The listing builds one solid part. Answer for the finished solid, in the listing's coordinates (mm). Give positions to 0.01 mm unless a question says otherwise; leave off trailing zeros. Loops run counter-clockwise (first coordinate to the right, second up) from the corner with the lowest first, then second, coordinate; pieces in that order, holes last. Notation, with made-up numbers: M 62,67 L 82,67 A17 ccw 82,81 Z; hole C 26,16.25 d7. An arc over 180 degrees is marked long. One line per item, written item: value. Start each with the question number.
Q1. A cutting plane is placed at A-A, the plane y = 0. Determine the outline of the cut face in (x, z), and give its area (3 significant figures).
Q2. Flat-ended cylindrical pins translate along their axes: pin 1 (8 mm diameter, centred on x = 8.5, y = -2, fed in from -Z); pin 2 (1.8 mm diameter, centred on y = -1, z = -98, fed in from +X). Find the tip coordinate at first contact, or state that the pin passes through.
Q3. A cutting plane is placed at B-B, the plane z = -99. Determine the outline of the cut face in (x, y), and give its area (3 significant figures).
Q4. A cutting plane is placed at C-C, the plane x = 10. Determine the outline of the cut face in (y, z).
Q5. A cutting plane is placed at D-D, the plane z = -65.5. Determine the outline of the cut face in (x, y), and give its area (3 significant figures).
Q6. Consider L1, parallel to Y at x = 10, z = -50; L2, parallel to Y at x = 18.9, z = -99; L3, parallel to X at y = -0.5, z = -48. Determine where each line is inside the solid, lowest interval first.
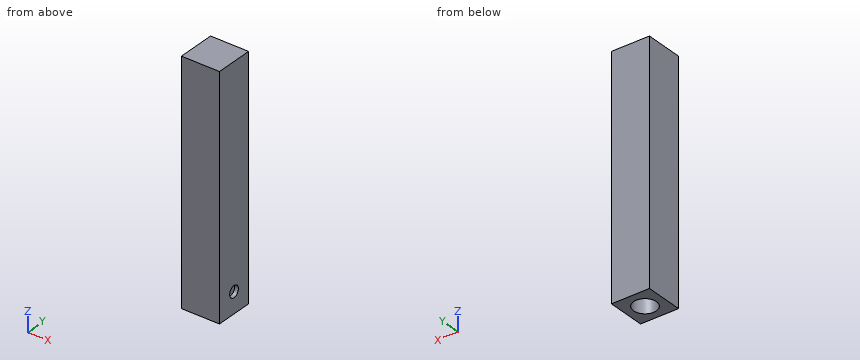
from build123d import *

# Parameters (mm, degrees)
EXTRUDE_1_DEPTH     = 20
SKETCH_2_R          = 6
CUT_EXTRUDE_1_DEPTH = 80
SKETCH_3_R          = 3
CUT_EXTRUDE_2_DEPTH = 2


with BuildPart() as part:
    # 草图1 → 凸台-拉伸1 (new body)
    with BuildSketch(Plane(origin=(0, 0, 0), x_dir=(0, 0, -1), z_dir=(1, 0, 0))):
        Polygon((-14.17593604, 10), (-14.175953417, -10), (110, -10), (110, 10), align=None)
    extrude(amount=EXTRUDE_1_DEPTH)

    # 草图2 → 切除-拉伸1 (cut)
    with BuildSketch(Plane(origin=(0, 0, -110), x_dir=(-1, 0, 0), z_dir=(0, 0, -1))):
        with Locations((-10, 0)):
            Circle(SKETCH_2_R)
    extrude(amount=-CUT_EXTRUDE_1_DEPTH, mode=Mode.SUBTRACT)

    # 草图3 → 切除-拉伸2 (cut)
    with BuildSketch(Plane(origin=(20, 0, 0), x_dir=(0, 0, -1), z_dir=(1, 0, 0))):
        with Locations((99, 0)):
            Circle(SKETCH_3_R)
    extrude(amount=-CUT_EXTRUDE_2_DEPTH, mode=Mode.SUBTRACT)


solid = part.part
Answer block:
1. outline: M 0,-110 L 4,-110 L 4,-30 L 16,-30 L 16,-110 L 20,-110 L 20,-102 L 18,-102 L 18,-96 L 20,-96 L 20,14.18 L 0,14.18 Z
1. area: 1,510 mm^2
2. pin 1: z = -110
2. pin 2: x = 18
3. outline: M 0,-10 L 20,-10 L 20,-3 L 18,-3 L 18,3 L 20,3 L 20,10 L 0,10 Z; hole C 10,0 d12
3. area: 275 mm^2
4. outline: M -10,-110 L -6,-110 L -6,-30 L 6,-30 L 6,-110 L 10,-110 L 10,14.18 L -10,14.18 Z
5. outline: M 0,-10 L 20,-10 L 20,10 L 0,10 Z; hole C 10,0 d12
5. area: 287 mm^2
6. L1: -10 to -6, 6 to 10
6. L2: -10 to -3, 3 to 10
6. L3: 0 to 4.02, 15.98 to 20
